Can you work these out from the model? Positions are in its coordinate system, mm. Face numbers are marked on the shaded views. A direction names the side the tool comes from. Give positions to 0.01 mm unless a question says otherwise; leave off trailing zeros. Write each loop counter-clockwise with the first axis right and the second up, starting at its lowest first coordinate (ties: lowest second). Pieces come first, ordered by that corner, then holes.
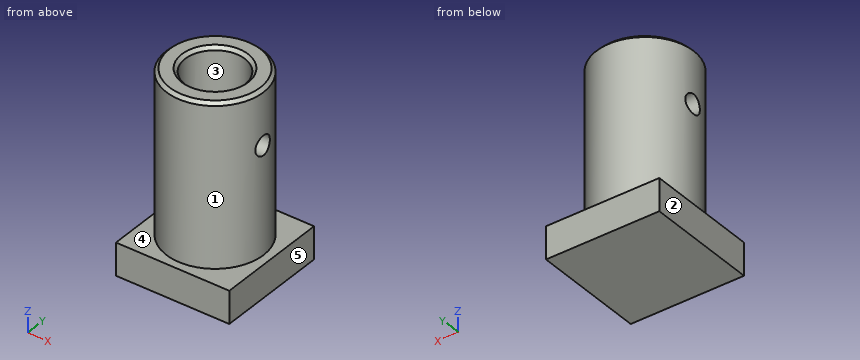
Autodesk Inventor part; units mm, degrees
ref_plane "YZ Plane" through (0, 0, 0) normal (1, 0, 0) x (0, 1, 0)
ref_plane "XZ Plane" through (0, 0, 0) normal (0, 1, 0) x (-1, 0, 0)
ref_plane "XY Plane" through (0, 0, 0) normal (0, 0, 1) x (1, 0, 0)
sketch "Эскиз1" plane through (0, 0, 0) normal (0, 0, 1) x (1, 0, 0)
  line L0 (17.5, -17.5) -> (-17.5, -17.5)
  line L1 (-17.5, -17.5) -> (-17.5, 17.5)
  line L2 (-17.5, 17.5) -> (17.5, 17.5)
  line L3 (17.5, 17.5) -> (17.5, -17.5)
  line L4 (17.5, -17.5) -> (-17.5, 17.5) construction
  line L5 (-17.5, -17.5) -> (17.5, 17.5) construction
  point P0 (0, 0)
  dimension "d0" = 35
  dimension "d1" = 35
extrude "Выдавливание1" add sketch "Эскиз1" against normal blind 10
sketch "Эскиз2" plane through (0, 0, 0) normal (0, 0, 1) x (1, 0, 0)
  circle A0 centre (0, 0) radius 15
  dimension "d4" = 30
extrude "Выдавливание2" add sketch "Эскиз2" along normal blind 50
sketch "Эскиз3" plane through (0, 0, 50) normal (0, 0, 1) x (1, 0, 0)
  point P0 (0, 0)
  point P1 (0, 0)
hole "Отверстие1" at (0, 0, 50) direction (0, 0, -1) diameter 18.5 depth 31 tip angle 120
sketch "Эскиз4" plane through (0, 0, 0) normal (1, 0, 0) x (0, 1, 0)
  circle A0 centre (0, 33) radius 3
  line L0 (0, -22) -> (0, 62)
  line L1 (17.5, 0) -> (-17.5, 0)
  line L2 (15, 50) -> (-15, 50)
  point P0 (0, 0)
  dimension "d14" = 6
  dimension "d15" = 17
extrude "Выдавливание3" cut sketch "Эскиз4" along normal mid plane 50
chamfer "Фаска1" distance 1 angle 45 2 edges at (-15, 0, 50) (0, 9.25, 50)
properties part number "Инж_граф_1"
(1) If we mould it in two halves opening along X, with no side actions, what happens to the marked faces 3, 4 and 5? For each: +X half, -X half, draft (parallel to the pull), parting line (faces both ways), or undercut.
Returned:
face 3: undercut
face 4: draft
face 5: +X half
(2) Imagine slicing it at A-A, the plane z = 33. Write out the boundary of the cut face in (x, y), plus the area to 3 significant figures.
Returned:
outline: (-14.7, -3) arc R15 ccw to (14.7, -3) - (8.75, -3) arc R9.25 cw to (-8.75, -3) - close; (-14.7, 3) - (-8.75, 3) arc R9.25 cw to (8.75, 3) - (14.7, 3) arc R15 ccw to start
area: 368 mm2
(3) Imagine slicing it at B-B, the plane y = -1.5. Give the number of separate pieces and of enclosed holes in the cut face, plus the area to 3 significant figures.
Returned:
separate pieces: 3
enclosed holes: 0
area: 1,170 mm2
(4) If I drill on L1, parallel to Z at x = 11.25, y = 0; L2, parallel to Y at x = 0, z = 28, over which ranges is the centre line in solid material (lowest first)?
Returned:
L1: z = -10 to 30, 36 to 50
L2: y = -15 to -9.25, 9.25 to 15
(5) Imagine slicing it at C-C, the plane z = 17.5. Write out the boundary of the cut face in (x, y), plus the area to 3 significant figures.
Returned:
outline: circle Ø30 at (0, 0); hole circle Ø13.3 at (0, 0)
area: 568 mm2
(6) For the marked faces 1 and 2, which set-ups out of +Z, -Z, +X, -X, +Y, -Y let a thin tool reach every point of the face, with its end or its side?
Returned:
face 1: +Z
face 2: +Z, -Z, -X, +Y, -Y
(7) Will these pins go through, and if not, where does the flat tip stop? P1, Ø8, axis at y = 0, z = 33, coming from the +X side; P2, Ø5.5, axis at y = 0, z = 33, coming from the +X side; P3, Ø1.5, axis at x = 1, z = 41.5, coming from the +Y side; P4, Ø6, axis at y = 5, z = 27, coming from the -X side.
Returned:
P1: stops at x = 15
P2: passes through
P3: stops at y = 15
P4: stops at x = -14.87
